Part model, mm, in its own coordinate system. A direction names the side the tool comes from. Coordinates: 2 decimals unless noted, no trailing zeros. Loops run counter-clockwise (first coordinate to the right, second up) from the corner with the lowest first, then second, coordinate; pieces in that order, holes last. Notation, with made-up numbers: (-25.5, -18) - (1.5, -18) arc R24 ccw to (1.5, -2) - close; hole circle Ø8 at (47, 29.5). An arc over 180 degrees is marked (long way). Use a Markdown table: item, result. Add a question column.
1. Wall check: probe 1 along Y at (x, z) = (-53, -4); probe 2 along Z at (x, y) = (4, -7.5) (3 decimals); probe 3 along Y at (x, z) = (-60, 6). Give the ranges that are in metal, low to high. Write a range as [from, to].
2. 3-axis set-ups, long thin cutter, end or side, ignore diameter. For faces 1 (the flat face through (-62, -8, -9.525)), 2 (the flat face through (-17.7, 49.9, 12.7)), 3 (the cylindrical face through (-26.69, 57.09, 11.45)), 4 (the flat face through (-53, -11.198, 0)), 5 (the flat face through (0.1, -0.05, 0.03)): which of +Z, -Z, +X, -X, +Y, -Y reach the whole face in a straight line?
3. Pull direction X, two halves, no side cores. Call faces 6 (the cylindrical face through (-67.963, -11.261, -5.662)), 7 (the flat face through (21, -15, 3.81)), 8 (the flat face through (-21, 5, -1.905)): pulls with the +X half, pulls with the -X half, needs draft (parallel to the pull), parting line crosses it, or undercut.
4. Band-saw the part on B-B, the plane z = -5. Give the cut face in (x, y).
5. Band-saw the part on A-A, the plane x = 21. Give the cut face in (y, z) (3 decimals), plus the area to 3 significant figures.
6. Drop flat-ended pins along their axis: pin 1 (12 mm diameter, centred on x = 20.02, y = -20.84, fed in from -Z) (3 decimals); pin 2 (9 mm diameter, centred on x = 20.02, y = -20.84, fed in from -Z); pin 3 (12 mm diameter, centred on x = 14, z = -4.5, fed in from -Y); pin 4 (4.5 mm diameter, centred on x = 23.5, y = -18, fed in from +Z). Give the stop position or say it passes through.
7. Band-saw the part on C-C, the plane x = -33.5. Give the cut face in (y, z) (3 decimals).
8. Band-saw the part on D-D, the plane y = 30. Give the cut face in (x, z) (3 decimals).
from build123d import *

# Parameters (mm, degrees)
F1_DEPTH        = 1.905
F2_R            = 9.34282
F3_DEPTH        = 12.7
F5_DEPTH        = 3.81
F6_R            = 18.50711
F7_DEPTH        = 9.525
F9_D            = 7.62
F9_DEPTH        = 101.6
F9_CBORE_D      = 13.97
F9_CBORE_DEPTH  = 2.54
F11_D           = 11.43
F11_DEPTH       = 101.6
F11_CBORE_D     = 15.24
F11_CBORE_DEPTH = 1.905
F13_DEPTH       = 19.051


with BuildPart() as f1:
    # F0 (on Top) → F1 (new body, symmetric)
    with BuildSketch(Plane.XY):
        with BuildLine():
            Line((-26.829338, 62.961267), (-69.205798, 13.704629))
            ThreePointArc((-69.205798, 13.704629), (-73.078408, -7.031412), (-56.99586, -20.681764))
            Line((-56.99586, -20.681764), (17.632922, -34.104249))
            ThreePointArc((17.632922, -34.104249), (33.078712, -24.160767), (24.254834, -8.049144))
            Line((24.254834, -8.049144), (-24.750318, 8.18019))
            Line((-24.750318, 8.18019), (-10.746106, 54.107821))
            ThreePointArc((-10.746106, 54.107821), (-15.194985, 65.061135), (-26.829338, 62.961267))
        make_face()
    extrude(amount=F1_DEPTH, both=True)

    # F2 (on Top) → F3 (join)
    with BuildSketch(Plane.XY):
        with Locations((-19.710172, 56.779236)):
            Circle(F2_R)
    extrude(amount=F3_DEPTH)

    # F4 (on face) → F5 (join)
    with BuildSketch(Plane.XY.offset(1.905)):
        with BuildLine():
            Line((24.254834, -8.049144), (23.161608, -7.687093))
            ThreePointArc((23.161608, -7.687093), (6.910327, -17.510066), (16.499491, -33.900394))
            Line((16.499491, -33.900394), (17.632922, -34.104249))
            ThreePointArc((17.632922, -34.104249), (33.078712, -24.160767), (24.254834, -8.049144))
        make_face()
    extrude(amount=F5_DEPTH)

    # F6 (on Top) → F7 (join, symmetric)
    with BuildSketch(Plane.XY):
        with Locations((-53.276106, 0)):
            Circle(F6_R)
    extrude(amount=F7_DEPTH, both=True)

    # F9
    with Locations(Plane.XY.offset(12.7)):
        with Locations((-19.710172, 56.779236)):
            CounterBoreHole(F9_D / 2, F9_CBORE_D / 2, F9_CBORE_DEPTH, depth=F9_DEPTH)

    # F11
    with Locations(Plane.XY.offset(5.715)):
        with Locations((20.018323, -20.841466)):
            CounterBoreHole(F11_D / 2, F11_CBORE_D / 2, F11_CBORE_DEPTH, depth=F11_DEPTH)

    # F12 (on face) → F13 (cut, through all)
    with BuildSketch(Plane.XY.offset(9.525)):
        Polygon((-46.810882, 11.198097), (-59.74133, 11.198097), (-66.206555, 0), (-59.74133, -11.198097), (-46.810882, -11.198097), (-40.345658, 0), align=None)
    extrude(amount=-F13_DEPTH, mode=Mode.SUBTRACT)


solid = f1.part
Geometry check:
| question | item | result |
|---|---|---|
| 1 | probe 1 | y = [-18.51, -11.2], [11.2, 18.51] |
| 1 | probe 2 | z = [-1.905, 1.905] |
| 1 | probe 3 | y = [-17.24, -10.75], [10.75, 17.24] |
| 2 | face 1 | -Z, +X, -X, +Y, -Y |
| 2 | face 2 | +Z, +X, -X, +Y, -Y |
| 2 | face 3 | +Z |
| 2 | face 4 | +Z, -Z |
| 2 | face 5 | +Z, -Z, +X |
| 3 | face 6 | parting line crosses it |
| 3 | face 7 | undercut |
| 3 | face 8 | needs draft |
| 4 | outline | circle Ø37.01 at (-53.28, 0); hole (-66.21, 0) - (-59.74, -11.2) - (-46.81, -11.2) - (-40.35, 0) - (-46.81, 11.2) - (-59.74, 11.2) - close |
| 5 | outline | (-34.281, -1.905) - (-26.472, -1.905) - (-26.472, 3.81) - (-28.398, 3.81) - (-28.398, 5.715) - (-34.281, 5.715) - close; (-15.211, -1.905) - (-6.971, -1.905) - (-6.971, 1.905) - (-7.352, 1.905) - (-7.352, 5.715) - (-13.285, 5.715) - (-13.285, 3.81) - (-15.211, 3.81) - close |
| 5 | area | 114 mm^2 |
| 6 | pin 1 | stops at z = -1.905 |
| 6 | pin 2 | passes through |
| 6 | pin 3 | stops at y = -34.3 |
| 6 | pin 4 | stops at z = 3.81 |
| 7 | outline | (-24.908, -1.905) - (55.208, -1.905) - (55.208, 1.905) - (-24.908, 1.905) - close |
| 8 | outline | (-55.187, -1.905) - (-18.097, -1.905) - (-18.097, 1.905) - (-55.187, 1.905) - close |
